Geometry check sheet. Reference: the model listing, model coordinates, mm. A direction names the side the tool comes from. Give positions to 0.01 mm unless a question says otherwise; leave off trailing zeros. Loops run counter-clockwise (first coordinate to the right, second up) from the corner with the lowest first, then second, coordinate; pieces in that order, holes last. Notation, with made-up numbers: (-34.75, 86) -> (-16.75, 86) arc R18 cw to (-16.75, 120) -> close; hole circle Ø1 at (53, -6). An arc over 180 degrees is marked (long way). Answer as a JSON object with one key per item and string values.
Autodesk Fusion 360 part; units mm, degrees
sketch "Sketch1" plane through (0, 0, 0) normal (0, 0, 1) x (1, 0, 0)
  line L0 (0, 121.92) -> (121.92, 121.92)
  line L1 (121.92, 121.92) -> (121.92, 0)
  line L2 (121.92, 0) -> (0, 0)
  line L3 (0, 0) -> (0, 121.92)
  line L4 (34.417, 69.469) -> (87.503, 69.469)
  line L5 (87.503, 69.469) -> (87.503, 52.451)
  line L6 (87.503, 52.451) -> (34.417, 52.451)
  line L7 (34.417, 52.451) -> (34.417, 69.469)
  dimension "d1" = 121.92
  dimension "d2" = 121.92
  dimension "d3" = 17.018
  dimension "d4" = 53.086
  dimension "d5" = 34.417
  dimension "d6" = 52.451
extrude "Extrude1" add sketch "Sketch1" along normal blind 102.616
sketch "Sketch2" plane through (0, 0, 0) normal (0, -1, 0) x (1, 0, 0)
  line L0 (0, 0) -> (121.92, 0)
  line L1 (121.92, 0) -> (121.92, 102.616)
  line L2 (121.92, 102.616) -> (0, 102.616)
  line L3 (0, 102.616) -> (0, 0)
  line L4 (-5.08, 102.616) -> (127, 102.616)
  line L5 (127, 102.616) -> (127, 97.536)
  line L6 (127, 97.536) -> (-5.08, 97.536)
  line L7 (-5.08, 97.536) -> (-5.08, 102.616)
  line L8 (-5.08, 0) -> (127, 0)
  line L9 (127, 0) -> (127, 5.08)
  line L10 (127, 5.08) -> (-5.08, 5.08)
  line L11 (-5.08, 5.08) -> (-5.08, 0)
  dimension "d9" = 5.08
  dimension "d10" = 132.08
  dimension "d11" = 5.08
  dimension "d12" = 132.08
  dimension "d13" = 5.08
  dimension "d14" = 5.08
extrude "Extrude2" add sketch "Sketch2" along normal blind 5.08 contours L0 L1 L3 L8 L10 | L3 L8 L10 L11 | L1 L8 L9 L10 | L3 L4 L6 L7 | L1 L2 L3 L4 L6 | L1 L4 L5 L6
sketch "Sketch3" plane through (121.92, 0, 0) normal (1, 0, 0) x (0, 1, 0)
  line L0 (0, 0) -> (121.92, 0)
  line L1 (121.92, 0) -> (121.92, 102.616)
  line L2 (121.92, 102.616) -> (0, 102.616)
  line L3 (0, 102.616) -> (0, 97.536)
  line L4 (0, 97.536) -> (0, 5.08)
  line L5 (0, 5.08) -> (0, 0)
  line L6 (0, 102.616) -> (121.92, 102.616)
  line L7 (121.92, 102.616) -> (121.92, 97.536)
  line L8 (121.92, 97.536) -> (0, 97.536)
  line L9 (0, 97.536) -> (0, 102.616)
  line L10 (0, 0) -> (121.92, 0)
  line L11 (121.92, 0) -> (121.92, 5.08)
  line L12 (121.92, 5.08) -> (0, 5.08)
  line L13 (0, 5.08) -> (0, 0)
  dimension "d17" = 5.08
  dimension "d18" = 5.08
extrude "Extrude3" add sketch "Sketch3" along normal blind 5.08 contours L0 L1 L5 L10 L11 L12 L13 | L1 L2 L3 L6 L7 L8 L9
sketch "Sketch4" plane through (0, 121.92, 0) normal (0, 1, 0) x (-1, 0, 0)
  line L0 (-127, 0) -> (0, 0)
  line L1 (0, 0) -> (0, 102.616)
  line L2 (0, 102.616) -> (-127, 102.616)
  line L3 (-127, 102.616) -> (-127, 97.536)
  line L4 (-127, 97.536) -> (-121.92, 97.536)
  line L5 (-121.92, 97.536) -> (-121.92, 5.08)
  line L6 (-121.92, 5.08) -> (-127, 5.08)
  line L7 (-127, 5.08) -> (-127, 0)
  line L8 (-127, 102.616) -> (5.08, 102.616)
  line L9 (5.08, 102.616) -> (5.08, 97.536)
  line L10 (5.08, 97.536) -> (-127, 97.536)
  line L11 (-127, 97.536) -> (-127, 102.616)
  line L12 (-127, 5.08) -> (5.08, 5.08)
  line L13 (5.08, 5.08) -> (5.08, 0)
  line L14 (5.08, 0) -> (-127, 0)
  line L15 (-127, 0) -> (-127, 5.08)
  dimension "d21" = 5.08
  dimension "d22" = 132.08
  dimension "d23" = 132.08
  dimension "d24" = 5.08
extrude "Extrude4" add sketch "Sketch4" along normal blind 5.08 contours L0 L1 L6 L7 L12 L14 L15 | L1 L12 L13 L14 | L1 L2 L3 L4 L8 L10 L11 | L1 L8 L9 L10
sketch "Sketch5" plane through (0, 0, 0) normal (-1, 0, 0) x (0, -1, 0)
  line L0 (-121.92, 0) -> (0, 0)
  line L1 (0, 0) -> (0, 5.08)
  line L2 (0, 5.08) -> (0, 97.536)
  line L3 (0, 97.536) -> (0, 102.616)
  line L4 (0, 102.616) -> (-121.92, 102.616)
  line L5 (-121.92, 102.616) -> (-121.92, 97.536)
  line L6 (-121.92, 97.536) -> (-121.92, 5.08)
  line L7 (-121.92, 5.08) -> (-121.92, 0)
  line L8 (-121.92, 102.616) -> (0, 102.616)
  line L9 (0, 102.616) -> (0, 97.536)
  line L10 (0, 97.536) -> (-121.92, 97.536)
  line L11 (-121.92, 97.536) -> (-121.92, 102.616)
  line L12 (-121.92, 5.08) -> (0, 5.08)
  line L13 (0, 5.08) -> (0, 0)
  line L14 (0, 0) -> (-121.92, 0)
  line L15 (-121.92, 0) -> (-121.92, 5.08)
  dimension "d27" = 5.08
  dimension "d28" = 5.08
extrude "Extrude5" add sketch "Sketch5" along normal blind 5.08 contours L0 L1 L7 L12 L13 L14 L15 | L3 L4 L5 L8 L9 L10 L11
sketch "Sketch6" plane through (0, 0, 0) normal (0, -1, 0) x (1, 0, 0)
  line L0 (0, 5.08) -> (121.92, 5.08)
  line L1 (121.92, 5.08) -> (121.92, 97.536)
  line L2 (121.92, 97.536) -> (0, 97.536)
  line L3 (0, 97.536) -> (0, 5.08)
  circle A0 centre (60.96, 51.308) radius 38.735
  line L4 (127, 102.616) -> (-5.08, 102.616)
  dimension "d31" = 77.47
  dimension "d32" = 51.308
  dimension "d33" = 60.96
extrude "Extrude6" cut sketch "Sketch6" against normal blind 44.704 contours A0
ref_plane "WorkPlane1" through (0, 60.96, 0) normal (0, 1, 0) x (0, 0, 1)
mirror "Mirror1" about plane through (0, 60.96, 0) normal (0, 1, 0) of "Extrude6"
sketch "Sketch7" plane through (0, 0, 102.616) normal (0, 0, 1) x (-1, 0, 0)
  line L0 (-87.503, -52.451) -> (-34.417, -52.451)
  line L1 (-34.417, -52.451) -> (-34.417, -69.469)
  line L2 (-34.417, -69.469) -> (-87.503, -69.469)
  line L3 (-87.503, -69.469) -> (-87.503, -52.451)
  line L4 (5.08, -127) -> (5.08, 5.08)
  line L5 (5.08, 5.08) -> (-127, 5.08)
  line L6 (-127, 5.08) -> (-127, -127)
  line L7 (-127, -127) -> (5.08, -127)
  line L8 (-57.023, -127) -> (-64.897, -127)
  line L9 (-64.897, -127) -> (-64.897, -82.296)
  line L10 (-64.897, -82.296) -> (-57.023, -82.296)
  line L11 (-57.023, -82.296) -> (-57.023, -127)
  line L12 (-33.7438, -60.96) -> (-1.1636, -60.96)
  line L13 (-64.897, -39.624) -> (-57.023, -39.624)
  line L14 (-57.023, -39.624) -> (-57.023, 5.08)
  line L15 (-64.897, 5.08) -> (-64.897, -39.624)
  line L16 (-57.023, 5.08) -> (-64.897, 5.08)
  dimension "d39" = 7.874
  dimension "d40" = 62.103
  dimension "d41" = 44.704
extrude "Extrude7" cut sketch "Sketch7" against normal blind 15.24 contours L7 L8 L9 L10 L11 | L5 L13 L14 L15 L16
sketch "Sketch8" plane through (0, 0, 102.616) normal (0, 0, 1) x (-1, 0, 0)
  line L0 (-87.503, -52.451) -> (-34.417, -52.451)
  line L1 (-34.417, -52.451) -> (-34.417, -69.469)
  line L2 (-34.417, -69.469) -> (-87.503, -69.469)
  line L3 (-87.503, -69.469) -> (-87.503, -52.451)
  line L4 (-64.897, -127) -> (-64.897, -82.296)
  line L5 (-64.897, -82.296) -> (-57.023, -82.296)
  line L6 (-57.023, -82.296) -> (-57.023, -127)
  line L7 (-57.023, -127) -> (5.08, -127)
  line L8 (5.08, -127) -> (5.08, 5.08)
  line L9 (5.08, 5.08) -> (-57.023, 5.08)
  line L10 (-57.023, 5.08) -> (-57.023, -39.624)
  line L11 (-57.023, -39.624) -> (-64.897, -39.624)
  line L12 (-64.897, -39.624) -> (-64.897, 5.08)
  line L13 (-64.897, 5.08) -> (-127, 5.08)
  line L14 (-127, 5.08) -> (-127, -127)
  line L15 (-127, -127) -> (-64.897, -127)
  circle A0 centre (-28.194, -60.96) radius 4.064
  circle A1 centre (-93.726, -60.96) radius 4.064
  dimension "d44" = 8.128
  dimension "d45" = 8.128
  dimension "d46" = 33.274
  dimension "d47" = 98.806
  dimension "d48" = 66.04
  dimension "d49" = 66.04
extrude "Extrude8" cut sketch "Sketch8" against normal blind 12.7 contours A0 | A1
thread "Thread1"
thread "Thread2"
fillet "Fillet1" radius 3.81 4 edges at (87.503, 69.469, 51.308) (34.417, 69.469, 51.308) (34.417, 52.451, 51.308) (87.503, 52.451, 51.308)
1) Section check D-D on x = 92. Record the cut outline in (y, z).
Geometry check:
{"outline": "(-5.08, 0) -> (127, 0) -> (127, 5.08) -> (121.92, 5.08) -> (121.92, 28.14) -> (77.22, 28.14) -> (77.22, 74.48) -> (121.92, 74.48) -> (121.92, 97.54) -> (127, 97.54) -> (127, 102.62) -> (64.64, 102.62) -> (64.64, 89.92) -> (57.28, 89.92) -> (57.28, 102.62) -> (-5.08, 102.62) -> (-5.08, 97.54) -> (0, 97.54) -> (0, 74.48) -> (44.7, 74.48) -> (44.7, 28.14) -> (0, 28.14) -> (0, 5.08) -> (-5.08, 5.08) -> close"}
2) Section check C-C on z = 34. Record the cut outline in (x, y), plus the area to 3 significant figures.
Geometry check:
{"outline": "(0, 0) -> (26.31, 0) -> (26.31, 44.7) -> (95.61, 44.7) -> (95.61, 0) -> (121.92, 0) -> (121.92, 121.92) -> (95.61, 121.92) -> (95.61, 77.22) -> (26.31, 77.22) -> (26.31, 121.92) -> (0, 121.92) -> close; hole (34.42, 56.26) arc R3.81 ccw to (38.23, 52.45) -> (83.69, 52.45) arc R3.81 ccw to (87.5, 56.26) -> (87.5, 65.66) arc R3.81 ccw to (83.69, 69.47) -> (38.23, 69.47) arc R3.81 ccw to (34.42, 65.66) -> close", "area": "7,780 mm2"}
3) Section check B-B on y = 60.96. Record the cut outline in (x, z), plus the area to 3 significant figures.
Geometry check:
{"outline": "(-5.08, 0) -> (34.42, 0) -> (34.42, 102.62) -> (32.26, 102.62) -> (32.26, 89.92) -> (24.13, 89.92) -> (24.13, 102.62) -> (-5.08, 102.62) -> (-5.08, 97.54) -> (0, 97.54) -> (0, 5.08) -> (-5.08, 5.08) -> close; (87.5, 0) -> (127, 0) -> (127, 5.08) -> (121.92, 5.08) -> (121.92, 97.54) -> (127, 97.54) -> (127, 102.62) -> (97.79, 102.62) -> (97.79, 89.92) -> (89.66, 89.92) -> (89.66, 102.62) -> (87.5, 102.62) -> close", "area": "6,960 mm2"}
4) Depth check by flat-ended pin: P1, Ø8, axis at x = 54, y = 93.5, coming from the -Z side; P2, Ø2, axis at x = 14, z = 42.5, coming from the -Y side; P3, Ø3, axis at y = 59, z = 48.5, coming from the +X side; P4, Ø2.5, axis at x = 60, z = 95, coming from the -Y side. Enter the tip coordinate at first touch or a pass-through.
Geometry check:
{"P1": "stops at z = 0", "P2": "stops at y = 0", "P3": "stops at x = 121.92", "P4": "stops at y = 39.62"}
5) Section check A-A on x = 60.96. Record the cut outline in (y, z).
Geometry check:
{"outline": "(-5.08, 0) -> (52.45, 0) -> (52.45, 102.62) -> (39.62, 102.62) -> (39.62, 90.04) -> (44.7, 90.04) -> (44.7, 12.57) -> (0, 12.57) -> (0, 5.08) -> (-5.08, 5.08) -> close; (69.47, 0) -> (127, 0) -> (127, 5.08) -> (121.92, 5.08) -> (121.92, 12.57) -> (77.22, 12.57) -> (77.22, 90.04) -> (82.3, 90.04) -> (82.3, 102.62) -> (69.47, 102.62) -> close"}
6) Tool access check on faces 1 (the face through (34.417, 61, 51)), 2 (the face through (121.92, 62, 51)), 3 (the face through (57.023, 104, 96)), 4 (the face through (96.74, 22.04, 36.47)). Record the directions out of +Z, -Z, +X, -X, +Y, -Y that give a thin tool (end or side, any length) a straight path to the whole face; none if there is none.
Geometry check:
{"face 1": "+Z, -Z", "face 2": "+X, +Y, -Y", "face 3": "+Z, +Y", "face 4": "-Y"}
7) Draft check along Y on faces 5 (the face through (60, 44.704, 52)), 6 (the face through (64.897, 17, 96)), 7 (the face through (87.503, 61, 51)). Enter one of: pulls with the +Y half, pulls with the -Y half, needs draft (parallel to the pull), parting line crosses it, or undercut.
Geometry check:
{"face 5": "pulls with the -Y half", "face 6": "needs draft", "face 7": "undercut"}
8) Material ranges on line 1 along X through (y, z) = (60.96, 99.5); line 2 along X through (y, z) = (64.5, 60); line 3 along X through (y, z) = (60, 95), recorded low to high. Write a range as from..to.
Geometry check:
{"line 1": "x = -5.08..24.13, 32.26..34.42, 87.5..89.66, 97.79..127", "line 2": "x = 0..34.42, 87.5..121.92", "line 3": "x = 0..24.25, 32.14..34.42, 87.5..89.78, 97.67..121.92"}
